```python
from build123d import *

# Parameters (mm, degrees)
BOSS_EXTRUDE1_DEPTH = 250
BOSS_EXTRUDE2_DEPTH = 0.8
SKETCH3_R           = 2
CUT_EXTRUDE2_DEPTH  = 8
FILLET1_R           = 5
SKETCH4_R           = 2
CUT_EXTRUDE3_DEPTH  = 8


with BuildPart() as part:
    # Sketch1 → Boss-Extrude1 (new body)
    with BuildSketch(Plane(origin=(0, 0, 0), x_dir=(1, 0, 0), z_dir=(0, 1, 0))):
        with BuildLine():
            Line((6.5, 9.5), (6.5, -20))
            Line((6.5, -20), (-20, -20))
            Line((-20, -20), (-20, 20))
            Line((-20, 20), (13, 20))
            Line((13, 20), (13, 19.6))
            Line((13, 19.6), (9.125718415, 17.5))
            ThreePointArc((9.125718415, 17.5), (7.173215496, 13.709940534), (6.5, 9.5))
        make_face()
    extrude(amount=BOSS_EXTRUDE1_DEPTH)

    # Sketch2 → Boss-Extrude2 (add)
    with BuildSketch(Plane(origin=(0, 0, -20), x_dir=(-1, 0, 0), z_dir=(0, 0, -1))):
        with BuildLine():
            Line((20, 225), (20, 250))
            Line((20, 250), (-13, 250))
            Line((-13, 250), (-13, 240))
            ThreePointArc((-13, 240), (-8.606601718, 229.393398282), (2, 225))
            Line((2, 225), (20, 225))
        make_face()
        with BuildLine():
            Line((-13, 0), (-13, 10))
            ThreePointArc((-13, 10), (-8.606601718, 20.606601718), (2, 25))
            Line((2, 25), (20, 25))
            Line((20, 25), (20, 0))
            Line((20, 0), (-13, 0))
        make_face()
    extrude(amount=BOSS_EXTRUDE2_DEPTH)

    # Sketch3 → Cut-Extrude2 (cut)
    with BuildSketch(Plane.XZ):
        with Locations((-15, 15)):
            Circle(SKETCH3_R)
        with Locations((0, 15)):
            Circle(SKETCH3_R)
        with Locations((0, -15.8)):
            Circle(SKETCH3_R)
        with Locations((-15, -15.8)):
            Circle(SKETCH3_R)
    cut_extrude2 = extrude(amount=-CUT_EXTRUDE2_DEPTH, mode=Mode.SUBTRACT)

    # Mirror1: Cut-Extrude2 across plane
    add(cut_extrude2.mirror(Plane.ZX.offset(125)), mode=Mode.SUBTRACT)

    # Fillet1
    fillet1_edges = [part.edges().sort_by_distance(p)[0] for p in [
        (-20, 125, -20),
    ]]
    fillet(fillet1_edges, radius=FILLET1_R)

    # Sketch4 → Cut-Extrude3 (cut)
    with BuildSketch(Plane(origin=(0, 0, -20.8), x_dir=(-1, 0, 0), z_dir=(0, 0, -1))):
        with Locations((5, 240)):
            Circle(SKETCH4_R)
    cut_extrude3 = extrude(amount=-CUT_EXTRUDE3_DEPTH, mode=Mode.SUBTRACT)

    # Mirror2: Cut-Extrude3 across plane
    add(cut_extrude3.mirror(Plane.ZX.offset(125)), mode=Mode.SUBTRACT)


solid = part.part
```
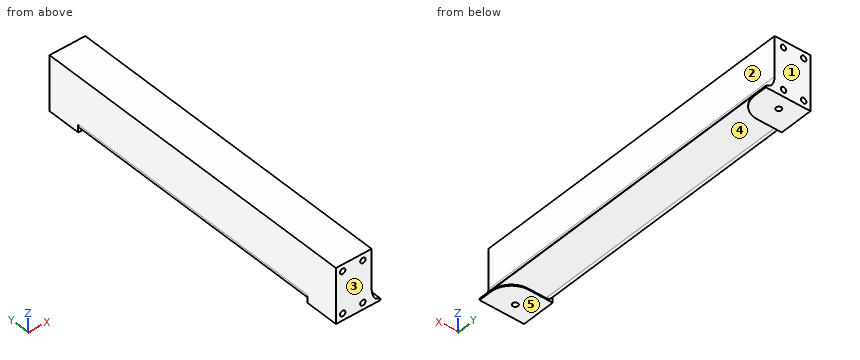
CAD build for the part. Positions are in the model's coordinates, mm. Face numbers are marked on the shaded views. A direction names the side the tool comes from. Round coordinates to 2 decimals unless told otherwise and drop trailing zeros. Order: outer loops, then holes, each group sorted by start corner. A loop starts at its lowest first (then second) coordinate and runs counter-clockwise, first axis right, second up. Notation, with made-up numbers: (-40, 30.25) - (-27, 30.25) arc R27 ccw to (-27, 57.25) - close; hole circle Ø9 at (17.5, 48). An arc over 180 degrees is marked (long way). Answer as CSV lines item,"result". Start each with the question number.
1. Saw through at B-B, the plane z = 8.5. Write the cut outline in (x, y), and give its area (4 significant figures).
2. Saw through at C-C, the plane y = 20.5. Write the cut outline in (x, z), and give its area (3 significant figures).
3. Pull direction Y, two halves, no side cores. Call the marked faces 3, 4 and 5: +Y half, -Y half, draft (parallel to the pull), parting line (faces both ways), or undercut.
4. Drill centre lines: L1, parallel to Z at x = -15, y = 2; L2, parallel to Z at x = -4.5, y = 65.5; L3, parallel to X at y = 82.5, z = 8. Where is each one in solid material? Low to high. Write a range as [from, to].
5. Tool access for the marked faces 1 and 2: list every direction of +Z, -Z, +X, -X, +Y, -Y with a clear straight run to the whole face (end or side of a thin tool).
6. Pin check, flat tips, straight feed: pin 1 (1.2 mm diameter, centred on x = -15.5, z = -16, fed in from +Y); pin 2 (3 mm diameter, centred on x = -5, y = 240, fed in from -Z); pin 3 (1.2 mm diameter, centred on x = 0.5, z = 14, fed in from -Y). Stop position of each tip, or through.
7. Saw through at A-A, the plane y = 103. Write the cut outline in (x, z), and give its area (3 significant figures).
Model answer:
1,outline,"(-20, 0) - (6.5, 0) - (6.5, 250) - (-20, 250) - close"
1,area,"6,625 mm²"
2,outline,"(-20, -20.8) - (8.71, -20.8) - (8.71, -20) - (13, -20) - (13, -19.6) - (9.13, -17.5) arc R13.5 cw to (6.5, -9.5) - (6.5, 20) - (-20, 20) - close"
2,area,"1,100 mm²"
3,face 3,"-Y half"
3,face 4,"undercut"
3,face 5,"draft"
4,L1,"z = [-20.8, -17.8], [-13.8, 13], [17, 20]"
4,L2,"z = [-20, 20]"
4,L3,"x = [-20, 6.5]"
5,face 1,"+Z, -Z, +X, -X, +Y"
5,face 2,"+Z, +X, +Y, -Y"
6,pin 1,"stops at y = 242"
6,pin 2,"stops at z = -12.8"
6,pin 3,"stops at y = 8"
7,outline,"(-20, -15) arc R5 ccw to (-15, -20) - (13, -20) - (13, -19.6) - (9.13, -17.5) arc R13.5 cw to (6.5, -9.5) - (6.5, 20) - (-20, 20) - close"
7,area,"1,070 mm²"
